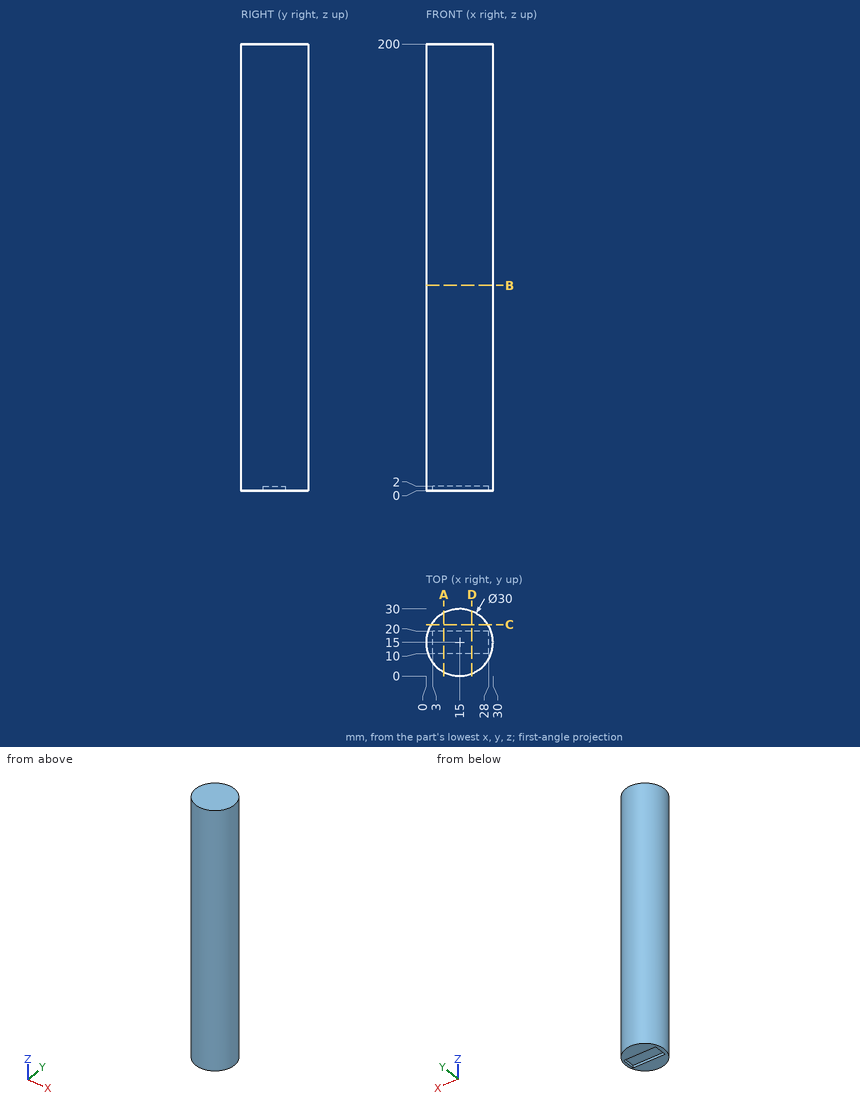
The drawing under review shows one solid part. Ordinate dimensions are in mm from its lowest x, y, z. Round coordinates to 2 decimals unless told otherwise and drop trailing zeros. Write each loop counter-clockwise with the first axis right and the second up, starting at its lowest first coordinate (ties: lowest second). Pieces come first, ordered by that corner, then holes.
(1) Insertion check: pin 1 (8 mm diameter, centred on x = 11.5, z = 131.5, fed in from -Y); pin 2 (1.5 mm diameter, centred on x = 13, z = 117.5, fed in from +Y); pin 3 (1 mm diameter, centred on y = 14, z = 1.5, fed in from -X); pin 4 (0.6 mm diameter, centred on x = 20.5, z = 1, fed in from -Y). Each pin has a flat end and moves straight along its axis. Give the tip position at first contact, or say it passes through.
(2) We need section D-D on x = 20.5. Give the boundary of the cut face in (y, z).
(3) We need section A-A on x = 8. Give the boundary of the cut face in (y, z).
(4) We need section B-B on z = 92. Give the boundary of the cut face in (x, y).
(5) We need section C-C on y = 23. Give the boundary of the cut face in (x, z), and give its area (3 significant figures).
(6) Wall thickness on L1, parallel to X at y = 14.75, z = 69; L2, parallel to X at y = 22.5, z = 181; L3, parallel to Z at x = 8.25, y = 14.75: over which ranges is each line inside the solid? List them lowest first.
Findings below:
1. pin 1: stops at y = 0
1. pin 2: stops at y = 29.95
1. pin 3: stops at x = 0.01
1. pin 4: stops at y = 0.93
2. outline: (1.04, 0) - (10, 0) - (10, 2) - (20, 2) - (20, 0) - (28.96, 0) - (28.96, 200) - (1.04, 200) - close
3. outline: (1.73, 0) - (10, 0) - (10, 2) - (20, 2) - (20, 0) - (28.27, 0) - (28.27, 200) - (1.73, 200) - close
4. outline: circle Ø30 at (15, 15)
5. outline: (2.31, 0) - (27.69, 0) - (27.69, 200) - (2.31, 200) - close
5. area: 5,080 mm2
6. L1: x = 0 to 30
6. L2: x = 2.01 to 27.99
6. L3: z = 2 to 200
